Could you check a few things on this drawing? It's one solid part, dimensions in mm from its lowest x, y, z. Give positions to 0.01 mm unless a question says otherwise; leave off trailing zeros. Write each loop counter-clockwise with the first axis right and the second up, starting at its lowest first coordinate (ties: lowest second). Pieces come first, ordered by that corner, then holes. Notation, with made-up numbers: (57.5, -21.75) -> (62.5, -21.75) arc R23 ccw to (62.5, -11.75) -> close; hole circle Ø2 at (46.25, -22). An arc over 180 degrees is marked (long way). Answer as CSV lines item,"result". Start each with the question number.
1. If we section it at B-B on y = 0.75: Write out the boundary of the cut face in (x, z) (1 decimal).
2. I need wall thicknesses on line 1 (X direction, y = 1.65, z = 99.5) (1 decimal); line 2 (Z direction, x = 175, y = 1.8) (1 decimal). Which ranges of each line are inside material? Lowest first, please. Write a range as [from, to].
3. If we section it at A-A on z = 103: Write out the boundary of the cut face in (x, y) (1 decimal).
4. If we section it at C-C on x = 85: Write out the boundary of the cut face in (y, z) (1 decimal), plus the area to 3 significant figures.
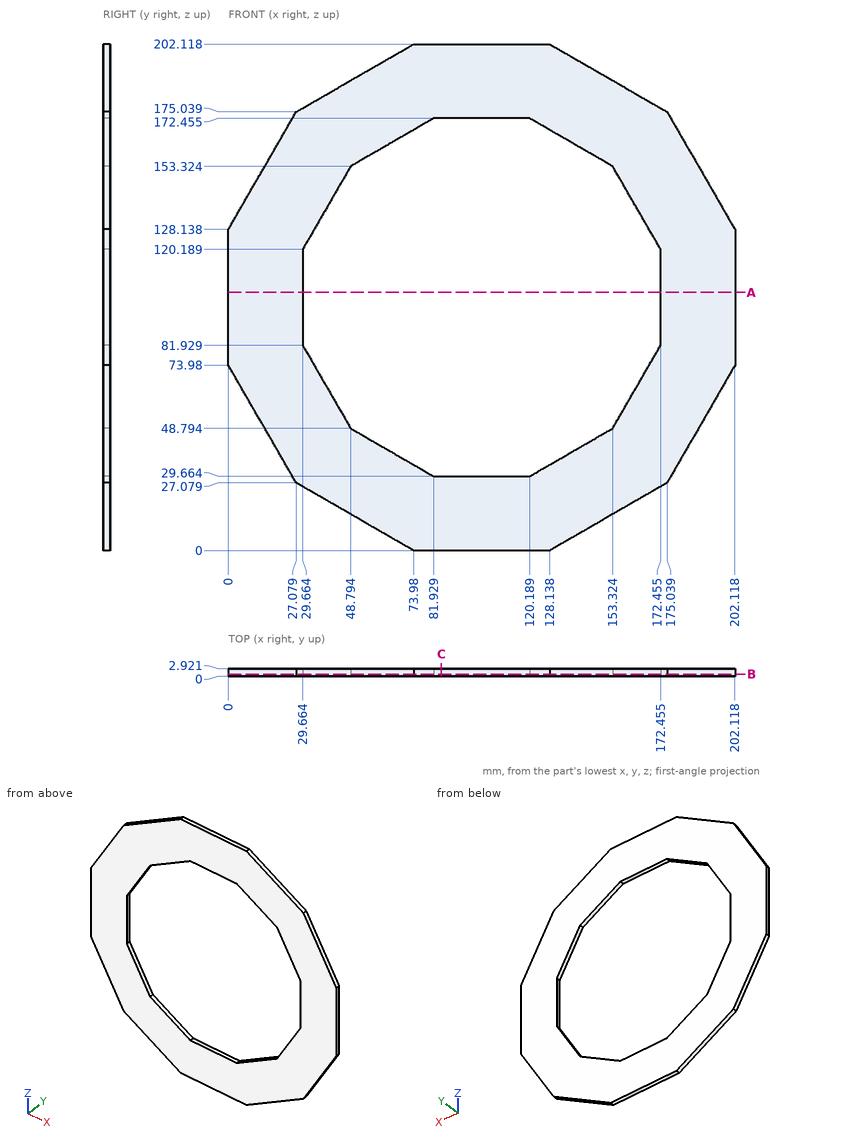
Computed values:
1,outline,"(0, 74) -> (27.1, 27.1) -> (74, 0) -> (128.1, 0) -> (175, 27.1) -> (202.1, 74) -> (202.1, 128.1) -> (175, 175) -> (128.1, 202.1) -> (74, 202.1) -> (27.1, 175) -> (0, 128.1) -> close; hole (29.7, 81.9) -> (48.8, 48.8) -> (81.9, 29.7) -> (120.2, 29.7) -> (153.3, 48.8) -> (172.5, 81.9) -> (172.5, 120.2) -> (153.3, 153.3) -> (120.2, 172.5) -> (81.9, 172.5) -> (48.8, 153.3) -> (29.7, 120.2) -> close"
2,line 1,"x = [0, 29.7], [172.5, 202.1]"
2,line 2,"z = [27.1, 175.1]"
3,outline,"(0, 0) -> (29.7, 0) -> (29.7, 2.9) -> (0, 2.9) -> close; (172.5, 0) -> (202.1, 0) -> (202.1, 2.9) -> (172.5, 2.9) -> close"
4,outline,"(0, 0) -> (2.9, 0) -> (2.9, 29.7) -> (0, 29.7) -> close; (0, 172.5) -> (2.9, 172.5) -> (2.9, 202.1) -> (0, 202.1) -> close"
4,area,"173 mm2"
